from build123d import *

# Parameters (mm, degrees)
SKETCH1_W           = 13
SKETCH1_H           = 13
SKETCH1_R           = 5
BOSS_EXTRUDE1_DEPTH = 13
CHAMFER1_SIZE       = 0.5


with BuildPart() as part:
    # Sketch1 → Boss-Extrude1 (new body)
    with BuildSketch(Plane.XY):
        Rectangle(SKETCH1_W, SKETCH1_H)
        with Locations(Location((0, 0, 0), (0, 0, 180))):
            Circle(SKETCH1_R, mode=Mode.SUBTRACT)
    extrude(amount=BOSS_EXTRUDE1_DEPTH)

    # Chamfer1
    chamfer1_edges = [part.edges().sort_by_distance(p)[0] for p in [
        (-6.5, 0, 13),
        (0, -6.5, 13),
        (6.5, 0, 13),
        (0, -6.5, 0),
        (-6.5, 0, 0),
        (0, 6.5, 0),
        (6.5, 0, 0),
        (6.5, -6.5, 6.5),
        (-6.5, -6.5, 6.5),
        (-6.5, 6.5, 6.5),
        (6.5, 6.5, 6.5),
        (0, 6.5, 13),
    ]]
    chamfer(chamfer1_edges, length=CHAMFER1_SIZE)


solid = part.part
Could you check a few things on this model? Use its own coordinates, in mm. Give positions to 0.01 mm unless a question says otherwise; leave off trailing zeros. Order: outer loops, then holes, each group sorted by start corner. A loop starts at its lowest first (then second) coordinate and runs counter-clockwise, first axis right, second up.
1. Suppose I cut it at A-A (y = 4). List the corners of the cut face in (x, z) for me.
2. Suppose I cut it at C-C (x = 0). List the corners of the cut face in (y, z) for me, plus the area to 3 significant figures.
3. We'd pull the mould along X, two halves only. Please class faces 1 (the cylindrical face through (5, 0, 6)), 2 (the flat face through (6.5, 0, 6)), 3 (the flat face through (5.2, 0.1, 13)): pulls with the +X half, pulls with the -X half, needs draft (parallel to the pull), parting line crosses it, or undercut.
4. Suppose I cut it at B-B (z = 5.75). List the corners of the cut face in (x, y) for me.
5. I need wall thicknesses on L1, parallel to Y at x = 0, z = 10.5; L2, parallel to X at y = -3.5, z = 7.5; L3, parallel to Y at x = -1.5, z = 9.75. Which ranges of each line are inside material? Lowest first, please.
Solved:
1. outline: (-6.5, 0.5) - (-6, 0) - (-3, 0) - (-3, 13) - (-6, 13) - (-6.5, 12.5) - close; (3, 0) - (6, 0) - (6.5, 0.5) - (6.5, 12.5) - (6, 13) - (3, 13) - close
2. outline: (-6.5, 0.5) - (-6, 0) - (-5, 0) - (-5, 13) - (-6, 13) - (-6.5, 12.5) - close; (5, 0) - (6, 0) - (6.5, 0.5) - (6.5, 12.5) - (6, 13) - (5, 13) - close
2. area: 38.5 mm2
3. face 1: undercut
3. face 2: pulls with the +X half
3. face 3: needs draft
4. outline: (-6.5, -6) - (-6, -6.5) - (6, -6.5) - (6.5, -6) - (6.5, 6) - (6, 6.5) - (-6, 6.5) - (-6.5, 6) - close; hole circle Ø10 at (0, 0)
5. L1: y = -6.5 to -5, 5 to 6.5
5. L2: x = -6.5 to -3.57, 3.57 to 6.5
5. L3: y = -6.5 to -4.77, 4.77 to 6.5
